Model file for the job. Use its own axes, mm. A direction names the side the tool comes from. Give positions to 0.01 mm unless a question says otherwise; leave off trailing zeros. Loops run counter-clockwise (first coordinate to the right, second up) from the corner with the lowest first, then second, coordinate; pieces in that order, holes last. Notation, with made-up numbers: M -24,3.25 L 22,3.25 A13 ccw 22,17.25 Z; hole C 50,-20 d11. An arc over 180 degrees is marked long. Answer in a Markdown table with one row per item.
```python
from build123d import *

# Parameters (mm, degrees)
SKETCH1_W                = 60
SKETCH1_H                = 95
BOSS_EXTRUDE1_DEPTH      = 1.3
SKETCH3_W                = 54.5
SKETCH3_H                = 53.1
BOSS_EXTRUDE2_DEPTH      = 39
SKETCH2_R                = 10.6
CUT_EXTRUDE1_DEPTH       = 4.7
SKETCH4_R                = 4.35
BOSS_EXTRUDE3_DEPTH      = 38
SKETCH5_R                = 17.2
BOSS_EXTRUDE4_DEPTH      = 34.4
FILLET1_R                = 17
M6_CLEARANCE_SLOT1_D     = 6.6
M5_CLEARANCE_SLOT1_DEPTH = 1.3
M5_CLEARANCE_SLOT2_DEPTH = 1.3
FILLET2_R                = 3


# Read off the part's stored shape, not the designer's step: M5 Clearance Slot1, M5 Clearance Slot2
with BuildPart() as part:
    # Sketch1 → Boss-Extrude1 (new body)
    with BuildSketch(Plane(origin=(0, 0, 0), x_dir=(1, 0, 0), z_dir=(0, 1, 0))):
        with Locations((30, 47.5)):
            Rectangle(SKETCH1_W, SKETCH1_H)
    extrude(amount=BOSS_EXTRUDE1_DEPTH)

    # Sketch3 → Boss-Extrude2 (add)
    with BuildSketch(Plane.XZ):
        with Locations((30, -47.5)):
            Rectangle(SKETCH3_W, SKETCH3_H)
    extrude(amount=BOSS_EXTRUDE2_DEPTH)

    # Sketch2 → Cut-Extrude1 (cut)
    with BuildSketch(Plane(origin=(0, 1.3, 0), x_dir=(1, 0, 0), z_dir=(0, 1, 0))):
        with Locations(Location((30, 47.5, 0), (0, 0, 270))):
            Circle(SKETCH2_R)
    extrude(amount=-CUT_EXTRUDE1_DEPTH, mode=Mode.SUBTRACT)

    # Sketch4 → Boss-Extrude3 (add)
    with BuildSketch(Plane(origin=(0, -3.4, 0), x_dir=(1, 0, 0), z_dir=(0, 1, 0))):
        with Locations(Location((30, 47.5, 0), (0, 0, 270))):
            Circle(SKETCH4_R)
    extrude(amount=BOSS_EXTRUDE3_DEPTH)

    # Sketch5 → Boss-Extrude4 (add)
    with BuildSketch(Plane(origin=(0, 34.6, 0), x_dir=(1, 0, 0), z_dir=(0, 1, 0))):
        with Locations(Location((30, 47.5, 0), (0, 0, 90))):
            Circle(SKETCH5_R)
    extrude(amount=BOSS_EXTRUDE4_DEPTH)

    # Fillet1
    # the kernel refuses this fillet: 17 mm, written as the material it takes off along each edge
    with BuildSketch(Plane(origin=(30, 34.6, -47.5), x_dir=(0, 0, -1), z_dir=(1, 0, 0))) as fillet1_piece_1:
        with BuildLine():
            CenterArc((0.2, 16.4856756), FILLET1_R, 284.129695419, 75.870304581)
            Line((4.35, 0), (4.433, -0.329713512))
            ThreePointArc((4.433, -0.329713512), (10.775, -0.34), (17.2, -0.34))
            Line((17.2, -0.34), (17.54, 0))
            Line((17.54, 0), (17.54, 16.4856756))
            Line((17.54, 16.4856756), (17.2, 16.4856756))
        make_face()
    revolve(axis=Axis((30, 34.6, -47.5), (0, 1, 0)), mode=Mode.SUBTRACT)
    with BuildSketch(Plane(origin=(30, 69, -47.5), x_dir=(0, 0, -1), z_dir=(1, 0, 0))) as fillet1_piece_2:
        with BuildLine():
            CenterArc((17.2 - FILLET1_R, -FILLET1_R), FILLET1_R, 0, 90)
            Line((17.2 - FILLET1_R, 0), (17.2 - FILLET1_R, FILLET1_R * 0.02))
            Line((17.2 - FILLET1_R, FILLET1_R * 0.02), (17.2, FILLET1_R * 0.02))
            Line((17.2, FILLET1_R * 0.02), (17.2 + FILLET1_R * 0.02, 0))
            Line((17.2 + FILLET1_R * 0.02, 0), (17.2 + FILLET1_R * 0.02, -FILLET1_R))
            Line((17.2 + FILLET1_R * 0.02, -FILLET1_R), (17.2, -FILLET1_R))
        make_face()
    revolve(axis=Axis((30, 69, -47.5), (0, 1, 0)), mode=Mode.SUBTRACT)

    # M6 Clearance Slot1 (through all)
    with Locations(Plane(origin=(0, 1.3, 0), x_dir=(1, 0, 0), z_dir=(0, 1, 0))):
        with Locations((30, 4.8), (30, 90.2)):
            Hole(M6_CLEARANCE_SLOT1_D / 2)

    # M5 Clearance Slot1 outline → M5 Clearance Slot1 (cut)
    with BuildSketch(Plane(origin=(0, 0, 0), x_dir=(1, 0, 0), z_dir=(0, 1, 0))):
        with BuildLine():
            Line((52.717157288, 3.25233406), (56.74766594, 7.282842712))
            ThreePointArc((56.74766594, 7.282842712), (56.74766594, 10.74766594), (53.282842712, 10.74766594))
            Line((53.282842712, 10.74766594), (49.25233406, 6.717157288))
            ThreePointArc((49.25233406, 6.717157288), (49.25233406, 3.25233406), (52.717157288, 3.25233406))
        make_face()
        with BuildLine():
            Line((6.717157288, 84.25233406), (10.74766594, 88.282842712))
            ThreePointArc((10.74766594, 88.282842712), (10.74766594, 91.74766594), (7.282842712, 91.74766594))
            Line((7.282842712, 91.74766594), (3.25233406, 87.717157288))
            ThreePointArc((3.25233406, 87.717157288), (3.25233406, 84.25233406), (6.717157288, 84.25233406))
        make_face()
    extrude(amount=M5_CLEARANCE_SLOT1_DEPTH, mode=Mode.SUBTRACT)

    # M5 Clearance Slot2 outline → M5 Clearance Slot2 (cut)
    with BuildSketch(Plane(origin=(0, 0, 0), x_dir=(1, 0, 0), z_dir=(0, 1, 0))):
        with BuildLine():
            Line((49.25233406, 88.282842712), (53.282842712, 84.25233406))
            ThreePointArc((53.282842712, 84.25233406), (56.74766594, 84.25233406), (56.74766594, 87.717157288))
            Line((56.74766594, 87.717157288), (52.717157288, 91.74766594))
            ThreePointArc((52.717157288, 91.74766594), (49.25233406, 91.74766594), (49.25233406, 88.282842712))
        make_face()
        with BuildLine():
            Line((3.25233406, 7.282842712), (7.282842712, 3.25233406))
            ThreePointArc((7.282842712, 3.25233406), (10.74766594, 3.25233406), (10.74766594, 6.717157288))
            Line((10.74766594, 6.717157288), (6.717157288, 10.74766594))
            ThreePointArc((6.717157288, 10.74766594), (3.25233406, 10.74766594), (3.25233406, 7.282842712))
        make_face()
    extrude(amount=M5_CLEARANCE_SLOT2_DEPTH, mode=Mode.SUBTRACT)

    # Fillet2
    fillet2_edges = [part.edges().sort_by_distance(p)[0] for p in [
        (0, 0.65, -95),
        (60, 0.65, -95),
        (60, 0.65, 0),
        (0, 0.65, 0),
    ]]
    fillet(fillet2_edges, radius=FILLET2_R)


solid = part.part
```
Q1. Saw through at C-C (z = -77). Give the cut face in (x, y), and give its area (3 significant figures).
Reported:
| item | result |
|---|---|
| outline | M 0,0 L 60,0 L 60,1.3 L 0,1.3 Z |
| area | 78.0 mm² |
Q2. Drop flat-ended pins along their axis: pin 1 (10.5 mm diameter, centred on x = 30, z = -90.2, fed in from -Y); pin 2 (2 mm diameter, centred on x = 18.5, y = -20.5, fed in from -Z); pin 3 (6 mm diameter, centred on x = 24, y = -23.5, fed in from +Z). Give the stop position or say it passes through.
Reported:
| item | result |
|---|---|
| pin 1 | y = 0 |
| pin 2 | z = -74.05 |
| pin 3 | z = -20.95 |
Q3. Saw through at B-B (x = 31.5). Give the number of separate pieces and of enclosed holes in the cut face, and give its area (3 significant figures).
Reported:
| item | result |
|---|---|
| separate pieces | 3 |
| enclosed holes | 0 |
| area | 3,330 mm² |
Q4. 3-axis set-ups, long thin cutter, end or side, ignore diameter. For faces 5 (the face through (57.25, -19, -48)), 6 (the face through (54.704, 0.641, -5.239)), 7 (the face through (30, -19, -20.95)), 8 (the face through (30.1, -3.4, -42.9)), 9 (the face through (30, -19, -74.05)): which of +Z, -Z, +X, -X, +Y, -Y reach the whole face in a straight line?
Reported:
| item | result |
|---|---|
| face 5 | +Z, -Z, +X, -Y |
| face 6 | +Y, -Y |
| face 7 | +Z, +X, -X, -Y |
| face 8 | none |
| face 9 | -Z, +X, -X, -Y |
Q5. Probe probe 1 along X at (y, z) = (-0.55, -47.5); probe 2 along Y at (x, z) = (12, -7); probe 3 along X at (y, z) = (-19, -23). List the from-to ranges inside material, lowest first.
Reported:
| item | result |
|---|---|
| probe 1 | 2.75 to 19.4, 25.65 to 34.35, 40.6 to 57.25 |
| probe 2 | 0 to 1.3 |
| probe 3 | 2.75 to 57.25 |
Q6. Mould opens along X. For faces 1 (the face through (10.785, 0.641, -91.709)), 2 (the face through (10.709, 0.641, -3.215)), 3 (the face through (2.75, -19, -48)), 4 (the face through (30, 1.3, -59)) say: released by +X, released by -X, zero draft, split by the parting line, or undercut.
Reported:
| item | result |
|---|---|
| face 1 | undercut |
| face 2 | undercut |
| face 3 | released by -X |
| face 4 | zero draft |
Q7. Saw through at A-A (z = -4.8). Give the cut face in (x, y).
Reported:
| item | result |
|---|---|
| outline | M 0,0 L 5.74,0 L 5.74,1.3 L 0,1.3 Z; M 11.46,0 L 26.7,0 L 26.7,1.3 L 11.46,1.3 Z; M 33.3,0 L 48.54,0 L 48.54,1.3 L 33.3,1.3 Z; M 54.26,0 L 60,0 L 60,1.3 L 54.26,1.3 Z |
